CAD build for the part. Positions are in the model's coordinates, mm. Face numbers are marked on the shaded views. A direction names the side the tool comes from. Give positions to 0.01 mm unless a question says otherwise; leave off trailing zeros. Write each loop counter-clockwise with the first axis right and the second up, starting at its lowest first coordinate (ties: lowest second). Pieces come first, ordered by that corner, then holes. Notation, with made-up numbers: (44.5, 11.5) - (61.5, 11.5) arc R24 cw to (61.5, 29.5) - close; hole circle Ø11 at (88.25, 75). An arc over 180 degrees is marked (long way). Answer as a JSON object with one key per item and string values.
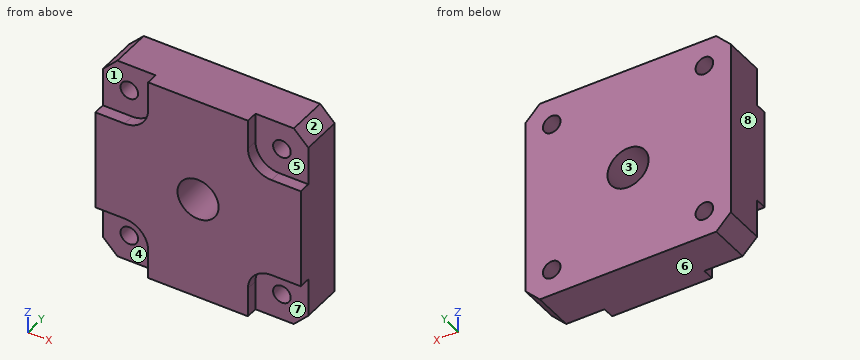
from build123d import *

# Parameters (mm, degrees)
SALIENTE_EXTRUIR1_DEPTH = 9
CROQUIS2_R              = 3.5
CORTAR_EXTRUIR1_DEPTH   = 51.309044912
CROQUIS3_R              = 1.5
CORTAR_EXTRUIR2_DEPTH   = 51.309044912
CUT_EXTRUDE1_DEPTH      = 2


with BuildPart() as part:
    # Croquis1 → Saliente-Extruir1 (new body)
    with BuildSketch(Plane(origin=(0, 0, 0), x_dir=(1, 0, 0), z_dir=(0, 1, 0))):
        Polygon((0, 2.473088065), (2.473088065, 0), (32.526911935, 0), (35, 2.473088065), (35, 32.526911935), (32.526911935, 35), (2.473088065, 35), (0, 32.526911935), align=None)
    extrude(amount=SALIENTE_EXTRUIR1_DEPTH)

    # Croquis2 → Cortar-Extruir1 (cut, through all)
    with BuildSketch(Plane(origin=(0, 9, 0), x_dir=(1, 0, 0), z_dir=(0, 1, 0))):
        with Locations(Location((17.5, 17.5, 0), (0, 0, 270))):
            Circle(CROQUIS2_R)
    extrude(amount=-CORTAR_EXTRUIR1_DEPTH, mode=Mode.SUBTRACT)

    # Croquis3 → Cortar-Extruir2 (cut, through all)
    with BuildSketch(Plane(origin=(0, 9, 0), x_dir=(1, 0, 0), z_dir=(0, 1, 0))):
        with Locations(Location((4.5, 30.5, 0), (0, 0, 270))):
            Circle(CROQUIS3_R)
        with Locations(Location((30.5, 30.5, 0), (0, 0, 270))):
            Circle(CROQUIS3_R)
        with Locations(Location((30.5, 4.5, 0), (0, 0, 270))):
            Circle(CROQUIS3_R)
        with Locations(Location((4.5, 4.5, 0), (0, 0, 270))):
            Circle(CROQUIS3_R)
    extrude(amount=-CORTAR_EXTRUIR2_DEPTH, mode=Mode.SUBTRACT)

    # Sketch1 → Cut-Extrude1 (cut)
    with BuildSketch(Plane.XZ):
        with BuildLine():
            Line((35, 0), (35, -9))
            Line((35, -9), (30, -9))
            ThreePointArc((30, -9), (27.171572875, -7.828427125), (26, -5))
            Line((26, -5), (26, 0))
            Line((26, 0), (35, 0))
        make_face()
        with BuildLine():
            Line((0, 0), (9, 0))
            Line((9, 0), (9, -5))
            ThreePointArc((9, -5), (7.828427125, -7.828427125), (5, -9))
            Line((5, -9), (0, -9))
            Line((0, -9), (0, 0))
        make_face()
        with BuildLine():
            Line((35, -35), (26, -35))
            Line((26, -35), (26, -30))
            ThreePointArc((26, -30), (27.171572875, -27.171572875), (30, -26))
            Line((30, -26), (35, -26))
            Line((35, -26), (35, -35))
        make_face()
        with BuildLine():
            Line((0, -35), (0, -26))
            Line((0, -26), (5, -26))
            ThreePointArc((5, -26), (7.828427125, -27.171572875), (9, -30))
            Line((9, -30), (9, -35))
            Line((9, -35), (0, -35))
        make_face()
    extrude(amount=-CUT_EXTRUDE1_DEPTH, mode=Mode.SUBTRACT)


solid = part.part
Item 1: Mould opens along X. For the marked faces 1, 2 and 3 say: +X half, -X half, draft (parallel to the pull), parting line (faces both ways), or undercut.
Entries:
{"face 1": "draft", "face 2": "+X half", "face 3": "undercut"}
Item 2: Which spindle directions (+Z, -Z, +X, -X, +Y, -Y) get a long thin tool onto all of the face, cutting with end or side? Do the marked faces 4, 5, 6, 7 and 8. Say none if no direction does.
Entries:
{"face 4": "-Z, -X, -Y", "face 5": "+Z, +X, -Y", "face 6": "-Z, +X, -X, +Y, -Y", "face 7": "-Z, +X, -Y", "face 8": "+Z, -Z, -X, +Y, -Y"}
Item 3: Cut at C-C (z = -4.5). Give the cut face in (x, y).
Entries:
{"outline": "(0, 2) - (3, 2) - (3, 9) - (0, 9) - close; (6, 2) - (9, 2) - (9, 0) - (26, 0) - (26, 2) - (29, 2) - (29, 9) - (6, 9) - close; (32, 2) - (35, 2) - (35, 9) - (32, 9) - close"}
Item 4: Probe line 1 (X direction, y = 4.75, z = -4.5); line 2 (X direction, y = 3.25, z = -17.5); line 3 (Z direction, x = 5.5, y = 8). List the from-to ranges inside material, lowest first. Write a range as from..to.
Entries:
{"line 1": "0..3, 6..29, 32..35", "line 2": "0..14, 21..35", "line 3": "-35..-31.62, -29.38..-5.62, -3.38..0"}
Item 5: Cut at B-B (y = 8.5). Give the cut face in (x, z), and give its area (3 significant figures).
Entries:
{"outline": "(0, -32.53) - (2.47, -35) - (32.53, -35) - (35, -32.53) - (35, -2.47) - (32.53, 0) - (2.47, 0) - (0, -2.47) - close; hole circle Ø3 at (4.5, -30.5); hole circle Ø3 at (4.5, -4.5); hole circle Ø7 at (17.5, -17.5); hole circle Ø3 at (30.5, -30.5); hole circle Ø3 at (30.5, -4.5)", "area": "1,150 mm2"}
Item 6: Cut at D-D (x = 31). Give the cut face in (y, z).
Entries:
{"outline": "(0, -26) - (2, -26) - (2, -29.09) - (9, -29.09) - (9, -5.91) - (2, -5.91) - (2, -9) - (0, -9) - close; (2, -35) - (9, -35) - (9, -31.91) - (2, -31.91) - close; (2, -3.09) - (9, -3.09) - (9, 0) - (2, 0) - close"}
Item 7: Flat gauge pins, fed straight in: P1, Ø0.6, axis at x = 33, y = 1, coming from the +Z side; P2, Ø7, axis at x = 3, z = -2.5, coming from the -Y side; P3, Ø1, axis at x = 33, y = 0.5, coming from the -Z side; P4, Ø4, axis at x = 17.5, z = -17.5, coming from the -Y side. Where does each tip first touch, or does it go through?
Entries:
{"P1": "z = -9", "P2": "y = 2", "P3": "z = -26", "P4": "through"}
Item 8: Cut at A-A (x = 17.5). Give the cut face in (y, z).
Entries:
{"outline": "(0, -35) - (9, -35) - (9, -21) - (0, -21) - close; (0, -14) - (9, -14) - (9, 0) - (0, 0) - close"}
